from build123d import *

# Parameters (mm, degrees)
F0_W     = 250
F0_H     = 230
F1_DEPTH = 5


with BuildPart() as f1:
    # F0 (on Top) → F1 (new body)
    with BuildSketch(Plane.XY):
        Rectangle(F0_W, F0_H)
        with BuildLine():
            ThreePointArc((-25, -80), (-30, -75), (-25, -70))
            Line((-25, -70), (25, -70))
            ThreePointArc((25, -70), (30, -75), (25, -80))
            Line((25, -80), (-25, -80))
        make_face(mode=Mode.SUBTRACT)
        with BuildLine():
            ThreePointArc((-25, -60), (-30, -55), (-25, -50))
            Line((-25, -50), (25, -50))
            ThreePointArc((25, -50), (30, -55), (25, -60))
            Line((25, -60), (-25, -60))
        make_face(mode=Mode.SUBTRACT)
    extrude(amount=F1_DEPTH)


solid = f1.part
The listing builds one solid part. Answer for the finished solid, in the listing's coordinates (mm). Give positions to 0.01 mm unless a question says otherwise; leave off trailing zeros. Order: outer loops, then holes, each group sorted by start corner. A loop starts at its lowest first (then second) coordinate and runs counter-clockwise, first axis right, second up. Notation, with made-up numbers: (17, 18.5) - (58, 18.5) arc R16 cw to (58, 44.5) - close; hole circle Ø1 at (-14, 66). An arc over 180 degrees is marked (long way). Answer as CSV lines item,"result".
Q1. A cutting plane is placed at A-A, the plane x = 10.5. Determine the outline of the cut face in (y, z).
Answer key:
outline,"(-115, 0) - (-80, 0) - (-80, 5) - (-115, 5) - close; (-70, 0) - (-60, 0) - (-60, 5) - (-70, 5) - close; (-50, 0) - (115, 0) - (115, 5) - (-50, 5) - close"
Q2. A cutting plane is placed at C-C, the plane z = 3.15. Determine the outline of the cut face in (x, y), and give its area (3 significant figures).
Answer key:
outline,"(-125, -115) - (125, -115) - (125, 115) - (-125, 115) - close; hole (-25, -80) - (25, -80) arc R5 ccw to (25, -70) - (-25, -70) arc R5 ccw to start; hole (-25, -60) - (25, -60) arc R5 ccw to (25, -50) - (-25, -50) arc R5 ccw to start"
area,"56,300 mm^2"
Q3. A cutting plane is placed at B-B, the plane y = -75. Determine the outline of the cut face in (x, z).
Answer key:
outline,"(-125, 0) - (-30, 0) - (-30, 5) - (-125, 5) - close; (30, 0) - (125, 0) - (125, 5) - (30, 5) - close"
Q4. Straight lines are drawn through the part: L1, parallel to Y at x = 3, z = 1.2; L2, parallel to X at y = -71, z = 1.9. For each, find the intervals that lie inside material, in ascending order.
Answer key:
L1,"y = -115 to -80, -70 to -60, -50 to 115"
L2,"x = -125 to -28, 28 to 125"
